For this review, take the finished solid that the model builds, in its own axes (mm). A direction names the side the tool comes from. Round coordinates to 2 decimals unless told otherwise and drop trailing zeros. Loops run counter-clockwise (first coordinate to the right, second up) from the corner with the lowest first, then second, coordinate; pieces in that order, holes last.
1) Mouldability with a two-part tool opening along Y and no side actions: class faces 1 (the flat face through (1, -21, -12)), 2 (the flat face through (0, -106.5, -6)), 3 (the flat face through (13.5, -75, -5)), 4 (the cylindrical face through (-33.05, -21.26, -9.24)) as pulls with the +Y half, pulls with the -Y half, needs draft (parallel to the pull), parting line crosses it, or undercut.
2) Take a section at C-C (x = 0). State the section outline as (y, z) points, then the cut area to 3 significant figures.
3) Insertion check: pin 1 (1.8 mm diameter, centred on y = -75, z = -0.5, fed in from -X) (3 decimals); pin 2 (0.8 mm diameter, centred on y = -74.5, z = -1, fed in from +X) (3 decimals); pin 3 (5.5 mm diameter, centred on x = 30, y = -20, fed in from -Z). Each pin has a flat end and moves straight along its axis. Give the tip position at first contact, or say it passes through.
4) Wall thickness on L1, parallel to X at y = -73, z = -0.75 (3 decimals); L2, parallel to X at y = -19, z = -2.5; L3, parallel to X at y = -58.5, z = -4.5 (3 decimals): over which ranges is each line inside the solid? List them lowest first.
5) Take a section at B-B (y = -73). State the section outline as (x, z) points (3 decimals).
6) Take a section at D-D (z = -4.5). Give the number of separate pieces and of enclosed holes in the cut face, then the cut area to 3 significant figures.
7) Tool access review of faces 5 (the flat face through (50, -20, -6)), 6 (the flat face through (13, -60, -9)), 7 (the cylindrical face through (-27.523, -105.502, -5.916)), 8 (the flat face through (-13.5, -75, -5)), 9 (the flat face through (34, -20, -6.4)): name each direction out of +Z, -Z, +X, -X, +Y, -Y from which nothing blocks a thin tool from reaching the whole face with its end or side.
8) Take a section at A-A (z = -10.5). State the section outline as (x, y) points (3 decimals).
```python
from build123d import *

# Parameters (mm, degrees)
EXTRUDE_1_DEPTH             = 12
HOLE_WIZARD_M61_D           = 6.6
HOLE_WIZARD_M61_CBORE_D     = 11
HOLE_WIZARD_M61_CBORE_DEPTH = 6.4
SKETCH_4_W                  = 57.15
SKETCH_4_H                  = 61
CUT_EXTRUDE_1_DEPTH         = 3
CUT_EXTRUDE_2_DEPTH         = 1.6
CUT_EXTRUDE_3_DEPTH         = 119.111853766
HOLE_START                  = -9
HOLE_WIZARD_M42_DEPTH       = 9


# Read off the part's stored shape, not the designer's step: Прорезь с зазором M42
with BuildPart() as part:
    # Эскиз1 → Бобышка-Вытянуть1 (new body)
    with BuildSketch(Plane.XY):
        with BuildLine():
            Line((-50, 0), (50, 0))
            Line((50, 0), (50, -40))
            Line((50, -40), (28.575, -43))
            Line((28.575, -43), (28.575, -103))
            ThreePointArc((28.575, -103), (27.549873734, -105.474873734), (25.075, -106.5))
            Line((25.075, -106.5), (-25.075, -106.5))
            ThreePointArc((-25.075, -106.5), (-27.549873734, -105.474873734), (-28.575, -103))
            Line((-28.575, -103), (-28.575, -43))
            Line((-28.575, -43), (-50, -40))
            Line((-50, -40), (-50, 0))
        make_face()
    extrude(amount=-EXTRUDE_1_DEPTH)

    # Цековка для  винта с внутренним шестигранником M61 (through all)
    with Locations(Plane.XY):
        with Locations((-30, -20), (30, -20)):
            CounterBoreHole(HOLE_WIZARD_M61_D / 2, HOLE_WIZARD_M61_CBORE_D / 2, HOLE_WIZARD_M61_CBORE_DEPTH)

    # Эскиз4 → Вырез-Вытянуть1 (cut)
    with BuildSketch(Plane(origin=(0, 0, -12), x_dir=(-1, 0, 0), z_dir=(0, 0, -1))):
        with Locations((0, -73.5)):
            Rectangle(SKETCH_4_W, SKETCH_4_H)
    extrude(amount=-CUT_EXTRUDE_1_DEPTH, mode=Mode.SUBTRACT)

    # Эскиз12 → Вырез-Вытянуть2 (cut)
    with BuildSketch(Plane.XY):
        with BuildLine():
            Line((-19.05, -80), (-19.05, -70))
            ThreePointArc((-19.05, -70), (0, -50.95), (19.05, -70))
            Line((19.05, -70), (19.05, -80))
            ThreePointArc((19.05, -80), (0, -99.05), (-19.05, -80))
        make_face()
    extrude(amount=-CUT_EXTRUDE_2_DEPTH, mode=Mode.SUBTRACT)

    # Эскиз13 → Вырез-Вытянуть3 (cut, through all)
    with BuildSketch(Plane.XY.offset(-1.6)):
        with BuildLine():
            Line((-13.5, -80), (-13.5, -70))
            ThreePointArc((-13.5, -70), (0, -56.5), (13.5, -70))
            Line((13.5, -70), (13.5, -80))
            ThreePointArc((13.5, -80), (0, -93.5), (-13.5, -80))
        make_face()
    extrude(amount=-CUT_EXTRUDE_3_DEPTH, mode=Mode.SUBTRACT)

    # Прорезь с зазором M42 outline → Прорезь с зазором M42 (cut)
    with BuildSketch(Plane.XY.offset(HOLE_START)):
        with BuildLine():
            ThreePointArc((-21.32, -95.82), (-23.57, -93.57), (-25.82, -95.82))
            Line((-25.82, -95.82), (-25.82, -101.32))
            ThreePointArc((-25.82, -101.32), (-23.57, -103.57), (-21.32, -101.32))
            Line((-21.32, -101.32), (-21.32, -95.82))
        make_face()
        with BuildLine():
            ThreePointArc((-21.32, -48.68), (-23.57, -46.43), (-25.82, -48.68))
            Line((-25.82, -48.68), (-25.82, -54.18))
            ThreePointArc((-25.82, -54.18), (-23.57, -56.43), (-21.32, -54.18))
            Line((-21.32, -54.18), (-21.32, -48.68))
        make_face()
        with BuildLine():
            ThreePointArc((25.82, -95.82), (23.57, -93.57), (21.32, -95.82))
            Line((21.32, -95.82), (21.32, -101.32))
            ThreePointArc((21.32, -101.32), (23.57, -103.57), (25.82, -101.32))
            Line((25.82, -101.32), (25.82, -95.82))
        make_face()
        with BuildLine():
            ThreePointArc((25.82, -48.68), (23.57, -46.43), (21.32, -48.68))
            Line((21.32, -48.68), (21.32, -54.18))
            ThreePointArc((21.32, -54.18), (23.57, -56.43), (25.82, -54.18))
            Line((25.82, -54.18), (25.82, -48.68))
        make_face()
    extrude(amount=HOLE_WIZARD_M42_DEPTH, mode=Mode.SUBTRACT)


solid = part.part
```
Response:
1. face 1: needs draft
1. face 2: pulls with the -Y half
1. face 3: undercut
1. face 4: undercut
2. outline: (-106.5, -12) - (-104, -12) - (-104, -9) - (-93.5, -9) - (-93.5, -1.6) - (-99.05, -1.6) - (-99.05, 0) - (-106.5, 0) - close; (-56.5, -9) - (-43, -9) - (-43, -12) - (0, -12) - (0, 0) - (-50.95, 0) - (-50.95, -1.6) - (-56.5, -1.6) - close
2. area: 744 mm2
3. pin 1: stops at x = -28.575
3. pin 2: stops at x = 28.575
3. pin 3: passes through
4. L1: x = -28.575 to -19.05, 19.05 to 28.575
4. L2: x = -50 to -35.41, -24.59 to 24.59, 35.41 to 50
4. L3: x = -28.575 to -7.071, 7.071 to 28.575
5. outline: (-28.575, -9) - (-13.5, -9) - (-13.5, -1.6) - (-19.05, -1.6) - (-19.05, 0) - (-28.575, 0) - close; (13.5, -9) - (28.575, -9) - (28.575, 0) - (19.05, 0) - (19.05, -1.6) - (13.5, -1.6) - close
6. separate pieces: 1
6. enclosed holes: 7
6. area: 6,660 mm2
7. face 5: +Z, -Z, +X, +Y, -Y
7. face 6: -Z, +X, -X
7. face 7: +Z, -Z, -X, -Y
7. face 8: +Z, -Z
7. face 9: +Z
8. outline: (-50, -40) - (-28.575, -43) - (28.575, -43) - (50, -40) - (50, 0) - (-50, 0) - close; (-28.429, -104) arc R3.5 ccw to (-25.075, -106.5) - (25.075, -106.5) arc R3.5 ccw to (28.429, -104) - close; hole circle Ø6.6 at (-30, -20); hole circle Ø6.6 at (30, -20)
